Can you work these out from the drawing? Everything is in mm from the part's minimum corner. Round coordinates to 2 decimals unless told otherwise and drop trailing zeros. Order: outer loops, then holes, each group sorted by start corner. A loop starts at its lowest first (then second) coordinate and runs counter-clockwise, first axis right, second up. Notation, with made-up numbers: (58.25, 69) -> (82.25, 69) arc R23 cw to (82.25, 79) -> close; hole circle Ø2 at (61.25, 11.25). An arc over 180 degrees is marked (long way). One line per item, written item: value.
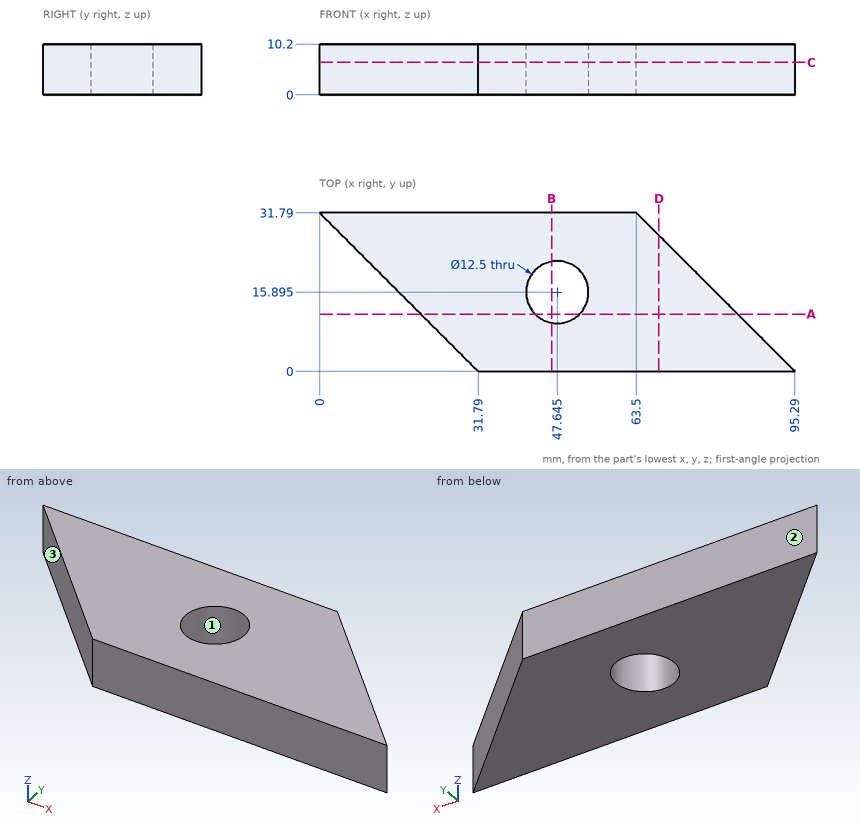
Q1. Will these pins go through, and if not, where does the flat tip stop? pin 1 Ø11 at (x, y) = (47.65, 15.9) entering from -Z; pin 2 Ø3 at (y, z) = (8.5, 2) entering from -X; pin 3 Ø1 at (y, z) = (13, 7) entering from +X.
Answers below:
pin 1: through
pin 2: x = 21.79
pin 3: x = 82.79
Q2. I want a section at B-B on x = 46.5. List the corners of the cut face in (y, z) for me, plus the area to 3 significant figures.
Answers below:
outline: (0, 0) -> (9.75, 0) -> (9.75, 10.2) -> (0, 10.2) -> close; (22.04, 0) -> (31.79, 0) -> (31.79, 10.2) -> (22.04, 10.2) -> close
area: 199 mm^2
Q3. I want a section at D-D on x = 68. List the corners of the cut face in (y, z) for me, plus the area to 3 significant figures.
Answers below:
outline: (0, 0) -> (27.29, 0) -> (27.29, 10.2) -> (0, 10.2) -> close
area: 278 mm^2
Q4. I want a section at C-C on z = 6.5. List the corners of the cut face in (x, y) for me (3 decimals).
Answers below:
outline: (0, 31.79) -> (31.79, 0) -> (95.29, 0) -> (63.5, 31.79) -> close; hole circle Ø12.5 at (47.645, 15.895)
Q5. I want a section at A-A on y = 11.5. List the corners of the cut face in (x, z) for me.
Answers below:
outline: (20.29, 0) -> (43.2, 0) -> (43.2, 10.2) -> (20.29, 10.2) -> close; (52.09, 0) -> (83.79, 0) -> (83.79, 10.2) -> (52.09, 10.2) -> close
Q6. Please list where these lines run through material, in increasing order: line 1 along X through (y, z) = (17, 7.75); line 2 along X through (y, z) = (19, 2.5); line 3 along X through (y, z) = (29, 6.75).
Answers below:
line 1: 14.79 to 41.49, 53.8 to 78.29
line 2: 12.79 to 42.22, 53.07 to 76.29
line 3: 2.79 to 66.29
Q7. We'd pull the mould along Y, two halves only. Please class the marked faces 1, 2 and 3: released by +Y, released by -Y, zero draft, split by the parting line, or undercut.
Answers below:
face 1: undercut
face 2: released by +Y
face 3: released by -Y
